Here's the drawing with two shaded views (mm, measured from the low corner). I have some questions. Round coordinates to 2 decimals unless told otherwise and drop trailing zeros. Loops run counter-clockwise (first coordinate to the right, second up) from the corner with the lowest first, then second, coordinate; pieces in that order, holes last.
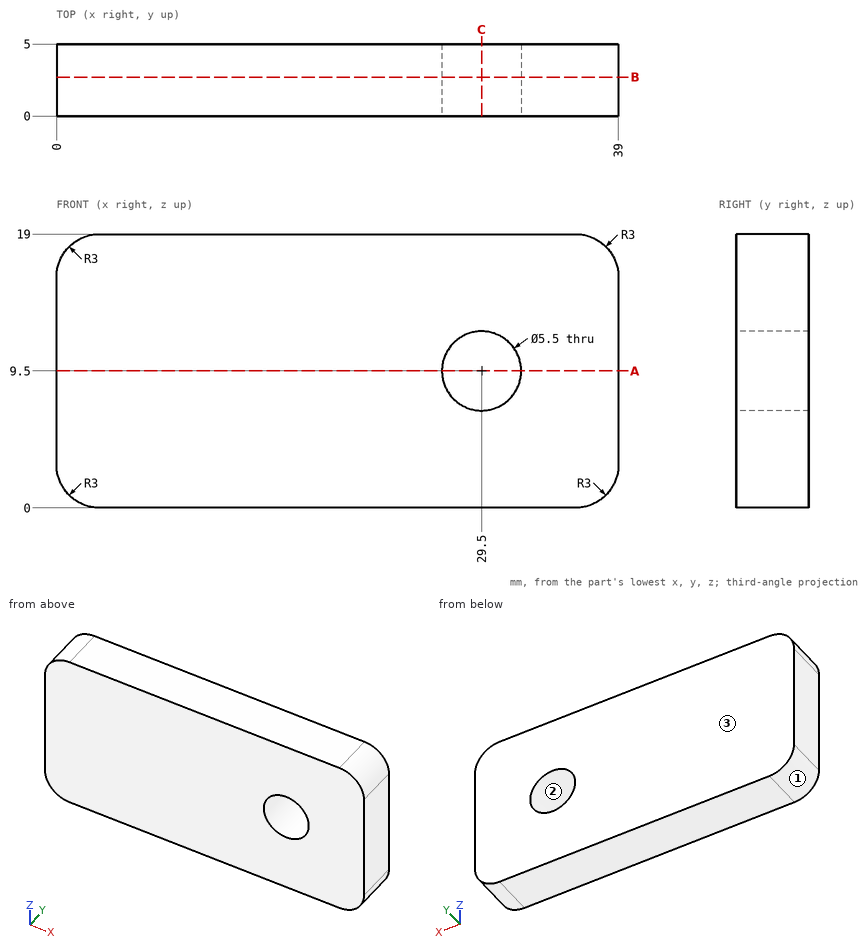
Item 1: We'd pull the mould along Z, two halves only. Please class the marked faces 1, 2 and 3: released by +Z, released by -Z, zero draft, split by the parting line, or undercut.
Results list:
face 1: released by -Z
face 2: undercut
face 3: zero draft
Item 2: If I drill on line 1 along Z through (x, y) = (29.5, 3.1); line 2 along X through (y, z) = (1.25, 8.25); line 3 along X through (y, z) = (3.9, 9), over which ranges is the centre line in solid material (lowest first)?
Results list:
line 1: z = 0 to 6.75, 12.25 to 19
line 2: x = 0 to 27.05, 31.95 to 39
line 3: x = 0 to 26.8, 32.2 to 39
Item 3: If we section it at C-C, the plane x = 29.5: Please give me the cut outline in (y, z), then the cut area to 3 significant figures.
Results list:
outline: (0, 0) - (5, 0) - (5, 6.75) - (0, 6.75) - close; (0, 12.25) - (5, 12.25) - (5, 19) - (0, 19) - close
area: 67.5 mm2
Item 4: If we section it at B-B, the plane y = 2.7: Please give me the cut outline in (x, z).
Results list:
outline: (0, 3) arc R3 ccw to (3, 0) - (36, 0) arc R3 ccw to (39, 3) - (39, 16) arc R3 ccw to (36, 19) - (3, 19) arc R3 ccw to (0, 16) - close; hole circle Ø5.5 at (29.5, 9.5)
Item 5: If we section it at A-A, the plane z = 9.5: Please give me the cut outline in (x, y).
Results list:
outline: (0, 0) - (26.75, 0) - (26.75, 5) - (0, 5) - close; (32.25, 0) - (39, 0) - (39, 5) - (32.25, 5) - close
